Source: CAD feature listing. Evaluate the final solid. Frame: model axes, mm. Face numbers are marked on the shaded views. A direction names the side the tool comes from. Round coordinates to 2 decimals unless told otherwise and drop trailing zeros. Order: outer loops, then holes, each group sorted by start corner. A loop starts at its lowest first (then second) coordinate and runs counter-clockwise, first axis right, second up. Notation, with made-up numbers: (4.25, 27) - (8.25, 27) arc R12 ccw to (8.25, 36) - close; hole circle Ø7 at (12, 39). An arc over 180 degrees is marked (long way). Use one line per item in the form item = value. Start each with the question number.
Q1. Set-up query: the marked faces 1 and 2. Return all of +Z, -Z, +X, -X, +Y, -Y with unobstructed straight access to the full face (end or side cutting, diameter ignored); none if empty.
Q2. Cut plane D-D, the plane x = -7. Return the cut outline in (y, z).
Q3. Pin query (flat end, axial travel): pin 1 Ø4.5 at (x, y) = (51.5, -6) entering from +Z; pin 2 Ø4 at (y, z) = (17.5, 12) entering from +X; pin 3 Ø6.5 at (x, y) = (12.5, 1.5) entering from +Z. Return the tip coordinate at first contact, or that it passes through.
Q4. Cut plane C-C, the plane y = -2.5. Return the cut outline in (x, z).
Q5. Cut plane A-A, the plane z = 3.5. Return the cut outline in (x, y).
Q6. Ray query, line 1 (Y direction, x = 7.5, z = 1.5); line 2 (X direction, y = -16, z = 18.5); line 3 (X direction, y = 0.5, z = 2.25). Return the intervals inside material, ascending. Write a range as [from, to].
Q7. Cut plane B-B, the plane z = 12.75. Return the cut outline in (x, y).
Q8. Draft query along X for the marked faces 3, 4 and 5. Return one class per face: released by +X, released by -X, zero draft, split by the parting line, or undercut.
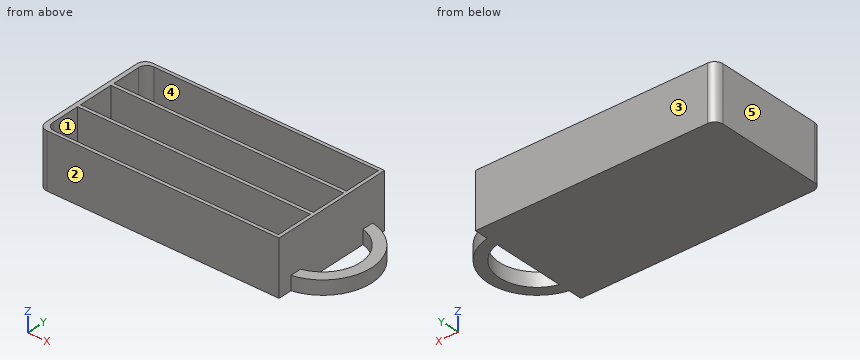
from build123d import *

# Parameters (mm, degrees)
SKETCH_1_W          = 86
SKETCH_1_H          = 44.4
EXTRUDE_1_DEPTH     = 19.6
EXTRUDE_2_DEPTH     = 5
SKETCH_3_W          = 83.2
SKETCH_3_H          = 13.4
SKETCH_3_H_2        = 12.8
CUT_EXTRUDE_1_DEPTH = 18.4
FILLET_1_R          = 3


with BuildPart() as part:
    # Эскиз1 → Бобышка-Вытянуть1 (new body)
    with BuildSketch(Plane.XY):
        Rectangle(SKETCH_1_W, SKETCH_1_H)
    extrude(amount=EXTRUDE_1_DEPTH)

    # Эскиз2 → Бобышка-Вытянуть2 (add)
    with BuildSketch(Plane.XY):
        with BuildLine():
            Line((43, 17.2), (43, 13.108775687))
            ThreePointArc((43, 13.108775687), (53.273546839, 0), (43, -13.108775687))
            Line((43, -13.108775687), (43, -17.2))
            ThreePointArc((43, -17.2), (57.273546839, 0), (43, 17.2))
        make_face()
    extrude(amount=EXTRUDE_2_DEPTH)

    # Эскиз3 → Вырез-Вытянуть1 (cut)
    with BuildSketch(Plane.XY.offset(19.6)):
        with Locations((0.2, 14.3)):
            Rectangle(SKETCH_3_W, SKETCH_3_H)
        with Locations((0.2, 0)):
            Rectangle(SKETCH_3_W, SKETCH_3_H_2)
        with Locations((0.2, -14.3)):
            Rectangle(SKETCH_3_W, SKETCH_3_H)
    extrude(amount=-CUT_EXTRUDE_1_DEPTH, mode=Mode.SUBTRACT)

    # Скругление1
    fillet_1_edges = [part.edges().sort_by_distance(p)[0] for p in [
        (-41.4, 21, 10.4),
        (-41.4, -21, 10.4),
        (-43, -22.2, 9.8),
        (-43, 22.2, 9.8),
    ]]
    fillet(fillet_1_edges, radius=FILLET_1_R)


solid = part.part
Completed:
q1.face_1 = +Z
q1.face_2 = +Z, -Z, +X, -X, -Y
q2.outline = (-22.2, 0) - (22.2, 0) - (22.2, 19.6) - (21, 19.6) - (21, 1.2) - (7.6, 1.2) - (7.6, 19.6) - (6.4, 19.6) - (6.4, 1.2) - (-6.4, 1.2) - (-6.4, 19.6) - (-7.6, 19.6) - (-7.6, 1.2) - (-21, 1.2) - (-21, 19.6) - (-22.2, 19.6) - close
q3.pin_1 = 5
q3.pin_2 = 43
q3.pin_3 = 1.2
q4.outline = (-43, 0) - (43, 0) - (43, 19.6) - (41.8, 19.6) - (41.8, 1.2) - (-41.4, 1.2) - (-41.4, 19.6) - (-43, 19.6) - close; (53.04, 0) - (57.09, 0) - (57.09, 5) - (53.04, 5) - close
q5.outline = (-43, -19.2) arc R3 ccw to (-40, -22.2) - (43, -22.2) - (43, -17.2) arc R17.5 ccw to (43, 17.2) - (43, 22.2) - (-40, 22.2) arc R3 ccw to (-43, 19.2) - close; hole (-41.4, -18) arc R3 ccw to (-38.4, -21) - (41.8, -21) - (41.8, -7.6) - (-41.4, -7.6) - close; hole (-41.4, -6.4) - (41.8, -6.4) - (41.8, 6.4) - (-41.4, 6.4) - close; hole (-41.4, 7.6) - (41.8, 7.6) - (41.8, 21) - (-38.4, 21) arc R3 ccw to (-41.4, 18) - close; hole (43, -13.11) arc R13.5 ccw to (43, 13.11) - close
q6.line_1 = [-22.2, -21], [-7.6, -6.4], [6.4, 7.6], [21, 22.2]
q6.line_2 = [-43, -41.4], [41.8, 43]
q6.line_3 = [-43, -41.4], [41.8, 43], [53.26, 57.27]
q7.outline = (-43, -19.2) arc R3 ccw to (-40, -22.2) - (43, -22.2) - (43, 22.2) - (-40, 22.2) arc R3 ccw to (-43, 19.2) - close; hole (-41.4, -18) arc R3 ccw to (-38.4, -21) - (41.8, -21) - (41.8, -7.6) - (-41.4, -7.6) - close; hole (-41.4, -6.4) - (41.8, -6.4) - (41.8, 6.4) - (-41.4, 6.4) - close; hole (-41.4, 7.6) - (41.8, 7.6) - (41.8, 21) - (-38.4, 21) arc R3 ccw to (-41.4, 18) - close
q8.face_3 = zero draft
q8.face_4 = undercut
q8.face_5 = released by -X
